```python
from build123d import *

# Parameters (mm, degrees)
F1_DEPTH      = 4
F1_DEPTH_BACK = 4
F2_COUNT      = 12


with BuildPart() as f1:
    # F0 (on Front) → F1 (new body, two sides)
    with BuildSketch(Plane.XZ) as f1_sk:
        Polygon((0, 0.75), (0, 0), (8.40777345, 0), (14.7618511692, 25.6429929286), (13.9891691904, 25.6429929286), (7.8209339859, 0.75), (7.5633733264, 0.75), (7.3573247987, 0.75), align=None)
    extrude(amount=F1_DEPTH)
    extrude(f1_sk.sketch, amount=-F1_DEPTH_BACK)

    # F2: F1 ×12 about axis
    f2_axis = Axis((0, 0, 1.0500000276), (0, 0, -1))


with BuildPart() as f1_1:
    add(f1.part)
    for i in range(1, F2_COUNT):
        add(f1.part.rotate(f2_axis, i * 360 / F2_COUNT))


solid = f1_1.part
```
Work out the finished part from the listing and answer in its coordinate system (mm). A direction names the side the tool comes from. Give positions to 0.01 mm unless a question says otherwise; leave off trailing zeros. Loops run counter-clockwise (first coordinate to the right, second up) from the corner with the lowest first, then second, coordinate; pieces in that order, holes last. Notation, with made-up numbers: (2.25, -32.5) - (48.25, -32.5) arc R12 cw to (48.25, -24.5) - close; hole circle Ø5 at (44, 41.25). An arc over 180 degrees is marked (long way). Use CSV: the item, a comma, the result in double quotes. Start each with the question number.
(1) Each of these flat-tipped pins is pushed along its axis until it touches: pin 1 (8 mm diameter, centred on y = -12.5, z = 14.5, fed in from -X); pin 2 (6 mm diameter, centred on x = 3.5, z = 3.5, fed in from -Y); pin 3 (6 mm diameter, centred on x = -8, z = 2.5, fed in from -Y). Where does it stop, or does it pass through?
(2) A tool of negligible diameter and unlimited length cuts with its end or side. For faces 4 (the face through (-1.5, 10.6, 8.1)), 5 (the face through (-6.636, -8.45, 8.133)), 6 (the face through (-5.429, 9.508, 13.371)), from which of +Z, -Z, +X, -X, +Y, -Y can it reach the whole face along a straight path? Write none if from no direction.
(3) Find section A-A, the plane x = -12.5. Determine the outline of the cut face in (y, z).
(4) Determine the mould class of faces 1 (the face through (0.055, 12.246, 15.491)), 2 (the face through (10, -4, 8)), 3 (the face through (8.45, 6.636, 8.133)) for opening direction X: released by +X, released by -X, zero draft, split by the parting line, or undercut.
(5) Find the intervals of material crossed by L1, parallel to X at y = -12.5, z = 17.5; L2, parallel to X at y = -6.5, z = 19.5; L3, parallel to Y at x = -7, z = 5.5, in increasing order.
Results found:
1,pin 1,"x = -9.56"
1,pin 2,"y = -10.5"
1,pin 3,"y = -8.29"
2,face 4,"-Z, +Y"
2,face 5,"-Z, -Y"
2,face 6,"+Z"
3,outline,"(-7.87, 25.64) - (-4, 17.83) - (-4, 16.51) - (-3.35, 16.51) - (-2.6, 15) - (-2.6, 16.51) - (2.6, 16.51) - (2.6, 15) - (3.35, 16.51) - (4, 16.51) - (4, 17.83) - (7.87, 25.64) - (6.33, 25.64) - (3.35, 19.63) - (-3.35, 19.63) - (-6.33, 25.64) - close"
4,face 1,"undercut"
4,face 2,"zero draft"
4,face 3,"released by +X"
5,L1,"-4 to 4"
5,L2,"-11.54 to -10.64, 10.64 to 11.54"
5,L3,"-7.42 to -5.87, 5.87 to 7.42"
